from build123d import *

# Parameters (mm, degrees)
F0_W     = 50.8
F0_H     = 25.4
F0_R     = 2.54
F0_W_2   = 38.1
F1_DEPTH = 5.08


with BuildPart() as f1:
    # F0 (on Right) → F1 (new body)
    with BuildSketch(Plane.YZ):
        with BuildLine():
            ThreePointArc((-615.5142915583, -231.0272213361), (-617.7461378856, -225.6390676635), (-623.1342915583, -223.4072213361))
            ThreePointArc((-623.1342915583, -223.4072213361), (-630.3184964873, -228.4872214272), (-627.9237613392, -236.9538881242))
            ThreePointArc((-627.9237613392, -236.9538881242), (-619.8503426953, -237.9032725187), (-615.5142915583, -231.0272213361))
        make_face()
        with BuildLine():
            Line((-603.4584249114, -347.8283836734), (-604.4899599765, -350.4072213361))
            Line((-604.4899599765, -350.4072213361), (-598.3495273174, -350.4072213361))
            ThreePointArc((-598.3495273174, -350.4072213361), (-601.2109621986, -349.7259681483), (-603.4584249114, -347.8283836734))
        make_face()
        with Locations((-261.5899599765, -236.1072213361)):
            Rectangle(F0_W, F0_H)
        with Locations((-242.5399599765, -229.7572213361)):
            Circle(F0_R, mode=Mode.SUBTRACT)
        with BuildLine():
            ThreePointArc((-645.5593421636, -337.7072213361), (-654.8692854334, -325.4680418144), (-669.1495020637, -331.1731248149))
            ThreePointArc((-669.1495020637, -331.1731248149), (-669.3108811021, -343.9644960696), (-658.2593421636, -350.4072213361))
            ThreePointArc((-658.2593421636, -350.4072213361), (-649.2790860425, -346.6874774572), (-645.5593421636, -337.7072213361))
        make_face()
        Polygon((-553.6899599765, -223.4072213361), (-604.4899599765, -223.4072213361), (-604.4899599765, -248.8072213361), (-563.8499599765, -248.8072213361), align=None)
        with Locations((-579.0899599765, -236.1072213361)):
            Circle(F0_R, mode=Mode.SUBTRACT)
        with Locations((-306.0399599765, -236.1072213361)):
            Rectangle(F0_W_2, F0_H)
        with Locations((-299.6899599765, -236.1072213361)):
            Circle(F0_R, mode=Mode.SUBTRACT)
        with BuildLine():
            Line((-546.6533227562, -248.8072213361), (-563.8499599765, -248.8072213361))
            Line((-563.8499599765, -248.8072213361), (-570.2366308991, -264.7738986426))
            ThreePointArc((-570.2366308991, -264.7738986426), (-560.8932947292, -253.1743138289), (-546.6533227562, -248.8072213361))
        make_face()
        with BuildLine():
            Line((-624.4345095354, -256.6481372677), (-604.4899599765, -223.4072213361))
            Line((-604.4899599765, -223.4072213361), (-623.1342915583, -223.4072213361))
            ThreePointArc((-623.1342915583, -223.4072213361), (-617.7461378856, -225.6390676635), (-615.5142915583, -231.0272213361))
            ThreePointArc((-615.5142915583, -231.0272213361), (-619.8503426953, -237.9032725187), (-627.9237613392, -236.9538881242))
            ThreePointArc((-627.9237613392, -236.9538881242), (-623.7505988619, -242.2393238717), (-622.262701352, -248.8072213361))
            ThreePointArc((-622.262701352, -248.8072213361), (-622.8156859424, -252.875289472), (-624.4345095354, -256.6481372677))
        make_face()
        with BuildLine():
            ThreePointArc((-592.8502662757, -340.8822208645), (-595.3537457832, -332.7190131593), (-594.0399626484, -324.2822280158))
            Line((-594.0399626484, -324.2822280158), (-599.4482722391, -337.8030019926))
            ThreePointArc((-599.4482722391, -337.8030019926), (-595.6640976039, -338.3030083357), (-592.8502662757, -340.8822208645))
        make_face()
        Polygon((-325.0899599765, -223.4072213361), (-553.6899599765, -223.4072213361), (-563.8499599765, -248.8072213361), (-546.6533227562, -248.8072213361), (-325.0899599765, -248.8072213361), align=None)
        with Locations((-337.7899599765, -236.1072213361)):
            Circle(F0_R, mode=Mode.SUBTRACT)
        with BuildLine():
            ThreePointArc((-592.8502662757, -340.8822208645), (-595.6640976039, -338.3030083357), (-599.4482722391, -337.8030019926))
            Line((-599.4482722391, -337.8030019926), (-603.4584249114, -347.8283836734))
            ThreePointArc((-603.4584249114, -347.8283836734), (-601.2109621986, -349.7259681483), (-598.3495273174, -350.4072213361))
            ThreePointArc((-598.3495273174, -350.4072213361), (-593.8593992569, -348.5473493967), (-591.9995273174, -344.0572213361))
            ThreePointArc((-591.9995273174, -344.0572213361), (-592.215898391, -342.4137201367), (-592.8502662757, -340.8822208645))
        make_face()
        with BuildLine():
            Line((-604.4899599765, -248.8072213361), (-604.4899599765, -223.4072213361))
            Line((-604.4899599765, -223.4072213361), (-624.4345095354, -256.6481372677))
            Line((-624.4345095354, -256.6481372677), (-669.1495020637, -331.1731248149))
            ThreePointArc((-669.1495020637, -331.1731248149), (-654.8692854334, -325.4680418144), (-645.5593421636, -337.7072213361))
            ThreePointArc((-645.5593421636, -337.7072213361), (-649.2790860425, -346.6874774572), (-658.2593421636, -350.4072213361))
            Line((-658.2593421636, -350.4072213361), (-604.4899599765, -350.4072213361))
            Line((-604.4899599765, -350.4072213361), (-603.4584249114, -347.8283836734))
            ThreePointArc((-603.4584249114, -347.8283836734), (-604.2453543046, -341.6988905413), (-599.4482722391, -337.8030019926))
            Line((-599.4482722391, -337.8030019926), (-594.0399626484, -324.2822280158))
            Line((-594.0399626484, -324.2822280158), (-570.2366308991, -264.7738986426))
            Line((-570.2366308991, -264.7738986426), (-563.8499599765, -248.8072213361))
            Line((-563.8499599765, -248.8072213361), (-604.4899599765, -248.8072213361))
        make_face()
        with Locations((-634.4372987192, -322.688178617)):
            Circle(F0_R, mode=Mode.SUBTRACT)
        with BuildLine():
            Line((-603.4584249114, -347.8283836734), (-599.4482722391, -337.8030019926))
            ThreePointArc((-599.4482722391, -337.8030019926), (-604.2453543046, -341.6988905413), (-603.4584249114, -347.8283836734))
        make_face()
    extrude(amount=F1_DEPTH)


solid = f1.part
Design review of the part built by this model. Coordinates are the model's own, in mm. Coordinates: 2 decimals unless noted, no trailing zeros. Loops run counter-clockwise (first coordinate to the right, second up) from the corner with the lowest first, then second, coordinate; pieces in that order, holes last. Notation, with made-up numbers: (43.5, 16) -> (64.5, 16) arc R11 ccw to (64.5, 34) -> close; hole circle Ø2 at (-28, 71.25). An arc over 180 degrees is marked (long way). Use a Markdown table: item, result. Add a question column.
Item 1: Wall thickness on L1, parallel to Y at x = 1.5, z = -230; L2, parallel to Z at x = 0.45, y = -458; L3, parallel to Z at x = 2.25, y = -636.5: over which ranges is each line inside the solid? List them lowest first. Write a range as from..to.
Item 2: We need section C-C, the plane z = -335. Write out the cut boundary in (x, y).
Item 3: Clearance check with flat-ended pins moving along their axes: P1, Ø4, axis at y = -337.79, z = -236.11, coming from the -X side; P2, Ø6.5, axis at y = -299.69, z = -236.11, coming from the -X side; P3, Ø2, axis at x = 2, z = -249, coming from the -Y side; P4, Ø1.5, axis at x = 4, z = -335.5, coming from the +Y side. State where each tip first meets the part, or that it passes through.
Item 4: We need section A-A, the plane x = 2.6. Write out the cut boundary in (y, z).
Item 5: We need section B-B, the plane y = -520.5. Write out the cut boundary in (x, z).
Numbers:
| question | item | result |
|---|---|---|
| 1 | L1 | y = -630.68..-245.07, -240.01..-236.19 |
| 1 | L2 | z = -248.81..-223.41 |
| 1 | L3 | z = -350.41..-324.17, -321.21..-276.76 |
| 2 | outline | (0, -670.67) -> (5.08, -670.67) -> (5.08, -595.05) -> (0, -595.05) -> close |
| 3 | P1 | passes through |
| 3 | P2 | stops at x = 0 |
| 3 | P3 | stops at y = -622.31 |
| 3 | P4 | stops at y = -594.76 |
| 4 | outline | (-669.15, -331.17) arc R12.7 ccw to (-658.26, -350.41) -> (-598.35, -350.41) arc R6.35 ccw to (-592.85, -340.88) arc R19.05 cw to (-594.04, -324.28) -> (-570.24, -264.77) arc R25.4 cw to (-546.65, -248.81) -> (-236.19, -248.81) -> (-236.19, -223.41) -> (-623.13, -223.41) arc R7.62 ccw to (-627.92, -236.95) arc R15.24 cw to (-624.43, -256.65) -> close; hole circle Ø5.08 at (-634.44, -322.69); hole circle Ø5.08 at (-579.09, -236.11); hole circle Ø5.08 at (-337.79, -236.11); hole circle Ø5.08 at (-299.69, -236.11); hole circle Ø5.08 at (-242.54, -229.76) |
| 5 | outline | (0, -248.81) -> (5.08, -248.81) -> (5.08, -223.41) -> (0, -223.41) -> close |
